Source: three-view drawing plus pictorial views. Frame: mm from the lowest corner of the part. Give positions to 0.01 mm unless a question says otherwise; leave off trailing zeros. Write each loop counter-clockwise with the first axis right and the second up, starting at its lowest first coordinate (ties: lowest second). Pieces come first, ordered by that corner, then holes. Notation, with made-up numbers: (-40, 25.5) -> (4, 25.5) arc R32 ccw to (4, 59.5) -> close; hole circle Ø3 at (38.25, 59). An arc over 180 degrees is marked (long way). Use a Markdown table: item, result. Add a question column.
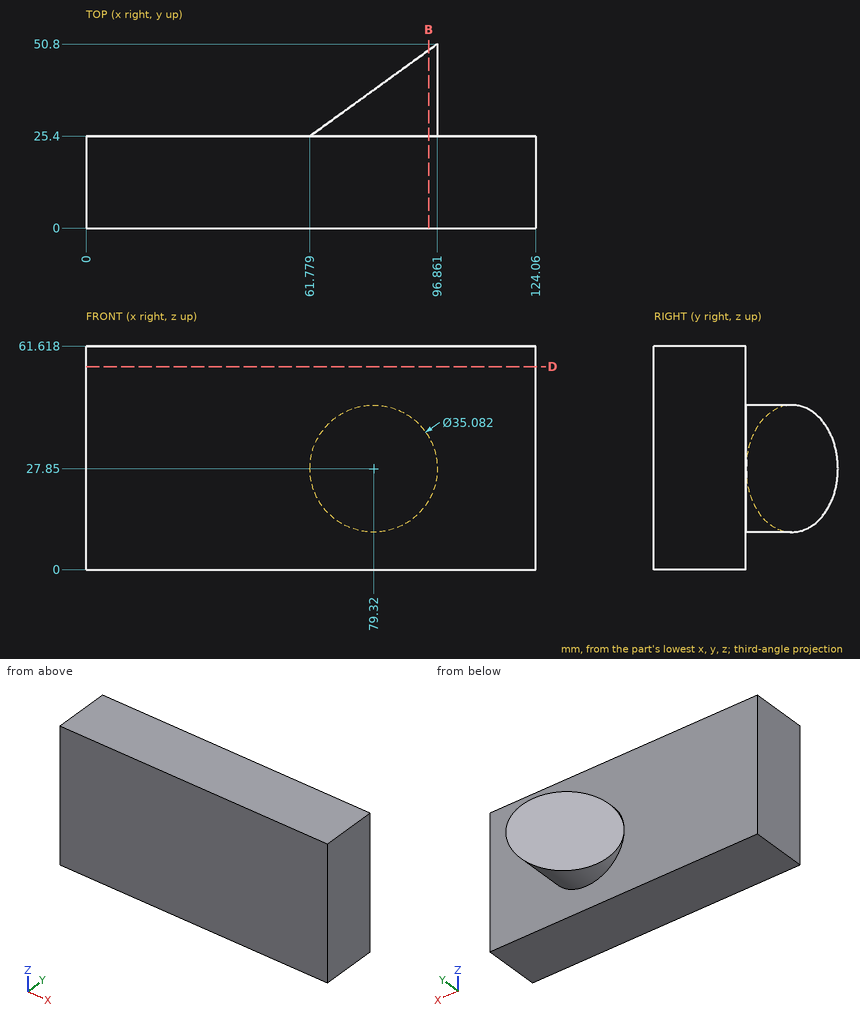
(1) Material intervals for L1, parallel to Y at x = 7, z = 41.5; L2, parallel to X at y = 42.5, z = 35.5 (1 decimal); L3, parallel to Y at x = 79, z = 21, sorted ascending.
(2) First-contact query: pin 1 Ø8 at (x, y) = (67.5, 35) entering from -Z; pin 2 Ø5 at (y, z) = (37.5, 46.5) entering from -X. Flat tips, straight axial feed; report the tip coordinate or a pass-through.
(3) Cut plane B-B on x = 94.5. Return the cut outline in (y, z), then the cut area to 3 significant figures.
(4) Cut plane D-D on z = 56. Return the cut outline in (x, y), then the cut area to 3 significant figures.
Output:
| question | item | result |
|---|---|---|
| 1 | L1 | 0 to 25.4 |
| 1 | L2 | 85.4 to 95.1 |
| 1 | L3 | 0 to 37.87 |
| 2 | pin 1 | through |
| 2 | pin 2 | x = 75.71 |
| 3 | outline | (0, 0) -> (25.4, 0) -> (25.4, 19.06) -> (49.09, 19.06) -> (49.09, 36.64) -> (25.4, 36.64) -> (25.4, 61.62) -> (0, 61.62) -> close |
| 3 | area | 1,980 mm^2 |
| 4 | outline | (0, 0) -> (124.06, 0) -> (124.06, 25.4) -> (0, 25.4) -> close |
| 4 | area | 3,150 mm^2 |
